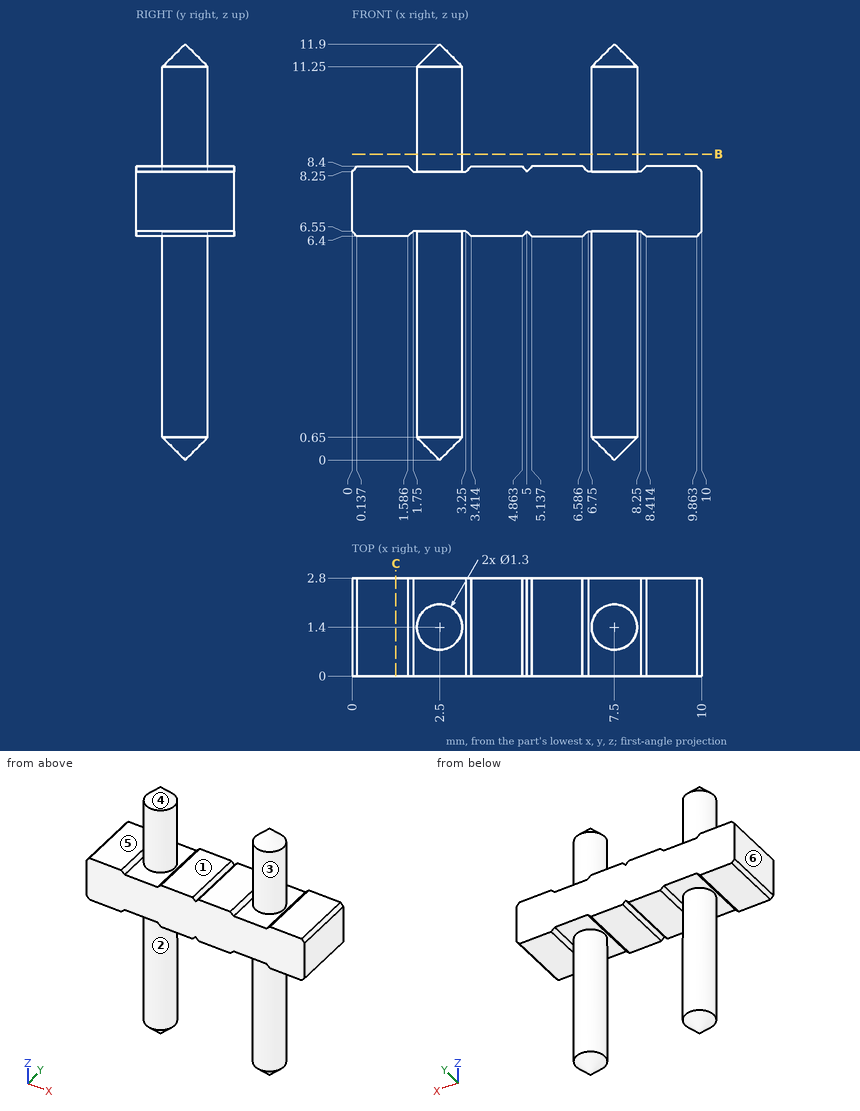
Verification items for this drawing (mm, ordinates from the low corner). A direction names the side the tool comes from. Give positions to 0.01 mm unless a question says otherwise; leave off trailing zeros. Loops run counter-clockwise (first coordinate to the right, second up) from the corner with the lowest first, then second, coordinate; pieces in that order, holes last. Notation, with made-up numbers: M -11,3 L 11,3 A32 ccw 11,39 Z; hole C 70.5,74.25 d9. An arc over 180 degrees is marked long. Answer as CSV lines item,"result".
Item 1: Depth check by flat-ended pin: P1, Ø1.6, axis at x = 4, y = 1, coming from the -Z side; P2, Ø1.5, axis at x = 3.5, z = 5.5, coming from the +Y side; P3, Ø1.2, axis at x = 4, y = 1, coming from the +Z side. Enter the tip coordinate at first touch or a pass-through.
Values:
P1,"stops at z = 6.4"
P2,"stops at y = 2"
P3,"stops at z = 8.4"
Item 2: Access from +Z, -Z, +X, -X, +Y, -Y to the whole of each face (thin tool, end or side, straight path). Record for the marked faces 1, 2 and 3.
Values:
face 1,"+Z, +Y, -Y"
face 2,"-Z"
face 3,"+Z"
Item 3: Release check for a two-part mould opening along X. For the marked faces 4, 5 and 6 record: pulls with the +X half, pulls with the -X half, needs draft (parallel to the pull), parting line crosses it, or undercut.
Values:
face 4,"undercut"
face 5,"needs draft"
face 6,"pulls with the -X half"
Item 4: Material ranges on line 1 (X direction, y = 1.35, z = 4); line 2 (Z direction, x = 4.5, y = 0.8); line 3 (X direction, y = 1, z = 5.25), recorded low to high.
Values:
line 1,"x = 1.85 to 3.15, 6.85 to 8.15"
line 2,"z = 6.4 to 8.4"
line 3,"x = 1.99 to 3.01, 6.99 to 8.01"
Item 5: Cross-section at C-C on x = 1.25. Record the cut outline in (y, z).
Values:
outline,"M 0,6.4 L 2.8,6.4 L 2.8,8.4 L 0,8.4 Z"
Item 6: Cross-section at B-B on z = 8.75. Record the cut outline in (x, y).
Values:
outline,"C 2.5,1.4 d1.3; C 7.5,1.4 d1.3"
